from build123d import *

# Parameters (mm, degrees)
F1_DEPTH = 8
F3_DEPTH = 10
F5_DEPTH = 9.9
F6_W     = 9
F6_H     = 8
F6_W_2   = 8
F7_DEPTH = 2
F6_R     = 1.3
F8_DEPTH = 6


with BuildPart() as f1:
    # F0 (on Top) → F1 (new body)
    with BuildSketch(Plane.XY):
        Polygon((28.5, -30), (-28.5, -30), (-36.985281, -21.514719), (-38.045942, -22.575379), (-30.62132, -30), (-33.166905, -32.545584), (-40.591526, -25.120963), (-41.652186, -26.181623), (-29.795584, -38.038225), (-24.257359, -32.5), (24.257359, -32.5), (29.795584, -38.038225), (41.652186, -26.181623), (40.591526, -25.120963), (33.166905, -32.545584), (30.62132, -30), (38.045942, -22.575379), (36.985281, -21.514719), align=None)
    extrude(amount=F1_DEPTH)

    # F2 (on face) → F3 (cut)
    with BuildSketch(Plane(origin=(33.916905, -33.916905, 0), x_dir=(0.707107, 0.707107, 0), z_dir=(0.707107, -0.707107, 0))):
        with BuildLine():
            ThreePointArc((7.671573, 4), (7.085786, 5.414214), (5.671573, 6))
            ThreePointArc((5.671573, 6), (3.671573, 4), (5.671573, 2))
            ThreePointArc((5.671573, 2), (7.085786, 2.585786), (7.671573, 4))
        make_face()
    extrude(amount=-F3_DEPTH, mode=Mode.SUBTRACT)

    # F4 (on face) → F5 (cut)
    with BuildSketch(Plane(origin=(-33.916905, -33.916905, 0), x_dir=(0.707107, -0.707107, 0), z_dir=(-0.707107, -0.707107, 0))):
        with BuildLine():
            ThreePointArc((-3.671573, 4), (-4.257359, 5.414214), (-5.671573, 6))
            ThreePointArc((-5.671573, 6), (-7.671573, 4), (-5.671573, 2))
            ThreePointArc((-5.671573, 2), (-4.257359, 2.585786), (-3.671573, 4))
        make_face()
    extrude(amount=-F5_DEPTH, mode=Mode.SUBTRACT)

    # F6 (on face) → F7 (join)
    with BuildSketch(Plane.XZ.offset(32.5)):
        with Locations((-16.757359, 4)):
            Rectangle(F6_W, F6_H)
        with Locations((10.257359, 4)):
            Rectangle(F6_W_2, F6_H)
    extrude(amount=F7_DEPTH)

    # F6 (on face) → F8 (join)
    with BuildSketch(Plane.XZ.offset(32.5)):
        with Locations((-8.757359, 5)):
            Circle(F6_R)
        with Locations((19.257359, 5)):
            Circle(F6_R)
    extrude(amount=F8_DEPTH)


solid = f1.part
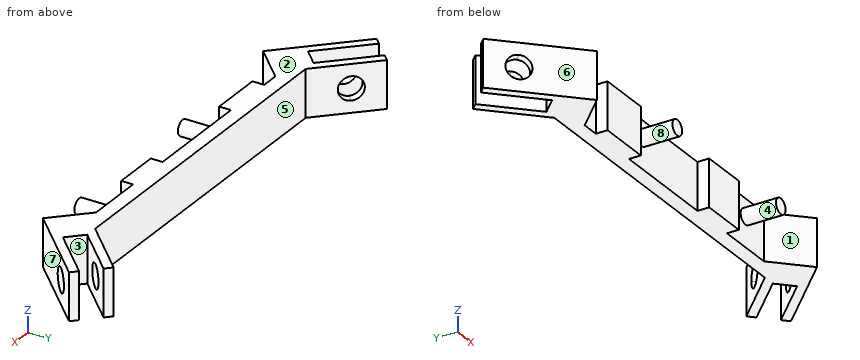
Input: part model. Units: mm. Frame: model coordinates. Face numbers are marked on the shaded views. A direction names the side the tool comes from. Give positions to 0.01 mm unless a question says otherwise; leave off trailing zeros. Loops run counter-clockwise (first coordinate to the right, second up) from the corner with the lowest first, then second, coordinate; pieces in that order, holes last. Notation, with made-up numbers: (47.25, 34.5) - (82.25, 34.5) arc R26 ccw to (82.25, 71.5) - close; hole circle Ø9 at (-21, 25). An arc over 180 degrees is marked (long way). Use CSV: the item, a comma, the result in double quotes. Start each with the question number.
Item 1: Mould query, pull axis X, two halves, no side actions, for the marked faces 6, 7 and 8. Classes: pulls with the +X half, pulls with the -X half, needs draft (parallel to the pull), parting line crosses it, or undercut.
Item 2: Section D-D on x = -1.5. Return loops of the section in (y, z).
Item 3: Section B-B on x = -13. Return loops of the section in (y, z).
Item 4: Contact query for flat-ended pins moving along their axis: P1, Ø1.6, axis at y = -33.5, z = 4, coming from the +X side; P2, Ø2.5, axis at x = -2, z = 6, coming from the -Y side; P3, Ø2, axis at y = -25, z = 1, coming from the -X side. Output: stop coordinate, or through.
Item 5: Line query: line 1 (X direction, y = -34.25, z = 7.5); line 2 (X direction, y = -27.75, z = 7); line 3 (X direction, y = -31.75, z = 3). Output: solid intervals per line, ascending.
Item 6: Reachability of the marked faces 1, 2, 3, 4 and 5 from +Z, -Z, +X, -X, +Y, -Y: full face, straight path, thin tool, end or side. Return the list, or none.
Item 7: Section C-C on z = 5. State how many separate pieces and enclosed holes the cut face has, then the cut area to 3 significant figures.
Item 8: Section A-A on y = -37.25. Return loops of the section in (x, z), then the cut area to 3 significant figures.
Ans:
1,face 6,"pulls with the -X half"
1,face 7,"pulls with the +X half"
1,face 8,"undercut"
2,outline,"(-32.5, 0) - (-30, 0) - (-30, 8) - (-32.5, 8) - close"
3,outline,"(-34.5, 0) - (-30, 0) - (-30, 8) - (-34.5, 8) - close"
4,P1,"stops at x = 35.13"
4,P2,"stops at y = -32.5"
4,P3,"stops at x = -41.47"
5,line 1,"x = -33.58 to -26.01, -21.26 to -12.26, 6.26 to 14.26, 26.01 to 33.58"
5,line 2,"x = -40.08 to -37.96, -32.87 to -30.75, 30.75 to 32.87, 37.96 to 40.08"
5,line 3,"x = -36.08 to -33.96, -32.37 to 32.37, 33.96 to 36.08"
6,face 1,"+Z, -Z, -Y"
6,face 2,"+Z, +X, -X, +Y, -Y"
6,face 3,"+Z, -Z"
6,face 4,"-Y"
6,face 5,"+Z, -Z, +Y"
7,separate pieces,"5"
7,enclosed holes,"0"
7,area,"328 mm2"
8,outline,"(-30.58, 0) - (-29.01, 0) - (-29.01, 8) - (-30.58, 8) - close; circle Ø2.6 at (-8.76, 5); circle Ø2.6 at (19.26, 5); (29.01, 0) - (30.58, 0) - (30.58, 8) - (29.01, 8) - close"
8,area,"35.8 mm2"
